from build123d import *

# Parameters (mm, degrees)
SKETCH_1_W             = 40
SKETCH_1_H             = 58
EXTRUDE_2_DEPTH        = 36
SKETCH_2_W             = 36
SKETCH_2_H             = 13
CUT_EXTRUDE_1_DEPTH    = 36
SKETCH_3_W             = 16
SKETCH_3_H             = 32
CUT_EXTRUDE_2_DEPTH    = 36
CUT_EXTRUDE_3_DEPTH    = 5
HOLE_WIZARD_M6_1_D     = 5
HOLE_WIZARD_M6_1_DEPTH = 15
HOLE_WIZARD_M6_1_TIP   = 1.502151548
CUT_EXTRUDE_START      = -36
SKETCH_8_W             = 12
SKETCH_8_H             = 32
CUT_EXTRUDE_4_DEPTH    = 36
FILLET_1_R             = 3
FILLET_2_R             = 5
SKETCH_9_W             = 36
SKETCH_9_H             = 32
CUT_EXTRUDE_5_DEPTH    = 0.5


with BuildPart() as part:
    # 草图1 → 凸台-拉伸2 (new body)
    with BuildSketch(Plane.XY):
        with Locations((20, 29)):
            Rectangle(SKETCH_1_W, SKETCH_1_H)
    extrude(amount=EXTRUDE_2_DEPTH)

    # 草图2 → 切除-拉伸1 (cut)
    with BuildSketch(Plane.ZY):
        with Locations((18, 51.5)):
            Rectangle(SKETCH_2_W, SKETCH_2_H)
        with Locations((18, 6.5)):
            Rectangle(SKETCH_2_W, SKETCH_2_H)
    extrude(amount=-CUT_EXTRUDE_1_DEPTH, mode=Mode.SUBTRACT)

    # 草图3 → 切除-拉伸2 (cut)
    with BuildSketch(Plane.ZY):
        with Locations((28, 29)):
            Rectangle(SKETCH_3_W, SKETCH_3_H)
    extrude(amount=-CUT_EXTRUDE_2_DEPTH, mode=Mode.SUBTRACT)

    # 草图4 → 切除-拉伸3 (cut)
    with BuildSketch(Plane(origin=(40, 0, 0), x_dir=(0, 0, -1), z_dir=(1, 0, 0))):
        with BuildLine():
            Line((-29, 53.1), (-7, 53.1))
            ThreePointArc((-7, 53.1), (-4.9, 51), (-7, 48.9))
            Line((-7, 48.9), (-29, 48.9))
            ThreePointArc((-29, 48.9), (-31.1, 51), (-29, 53.1))
        make_face()
        with BuildLine():
            Line((-29, 9.1), (-7, 9.1))
            ThreePointArc((-7, 9.1), (-4.9, 7), (-7, 4.9))
            Line((-7, 4.9), (-29, 4.9))
            ThreePointArc((-29, 4.9), (-31.1, 7), (-29, 9.1))
        make_face()
    extrude(amount=-CUT_EXTRUDE_3_DEPTH, mode=Mode.SUBTRACT)

    # M6 螺纹孔1
    with Locations(Plane.XY.offset(20)):
        with Locations((26, 29), (8, 29)):
            Hole(HOLE_WIZARD_M6_1_D / 2, depth=HOLE_WIZARD_M6_1_DEPTH)
            with Locations((0, 0, -(HOLE_WIZARD_M6_1_DEPTH + HOLE_WIZARD_M6_1_TIP / 2))):  # 118° drill point
                Cone(0, HOLE_WIZARD_M6_1_D / 2, HOLE_WIZARD_M6_1_TIP, mode=Mode.SUBTRACT)

    # 草图8 → 切除-拉伸4 (cut)
    with BuildSketch(Plane.ZY.offset(CUT_EXTRUDE_START)):
        with Locations((6, 29)):
            Rectangle(SKETCH_8_W, SKETCH_8_H)
    extrude(amount=CUT_EXTRUDE_4_DEPTH, mode=Mode.SUBTRACT)

    # 圆角1
    fillet_1_edges = [part.edges().sort_by_distance(p)[0] for p in [
        (38, 58, 36),
        (38, 0, 0),
        (38, 0, 36),
        (38, 58, 0),
    ]]
    fillet(fillet_1_edges, radius=FILLET_1_R)

    # 圆角2
    fillet_2_edges = [part.edges().sort_by_distance(p)[0] for p in [
        (0, 45, 16),
        (0, 13, 16),
    ]]
    fillet(fillet_2_edges, radius=FILLET_2_R)

    # 草图9 → 切除-拉伸5 (cut)
    with BuildSketch(Plane(origin=(40, 0, 0), x_dir=(0, 0, -1), z_dir=(1, 0, 0))):
        with Locations((-18, 29)):
            Rectangle(SKETCH_9_W, SKETCH_9_H)
    extrude(amount=-CUT_EXTRUDE_5_DEPTH, mode=Mode.SUBTRACT)


solid = part.part
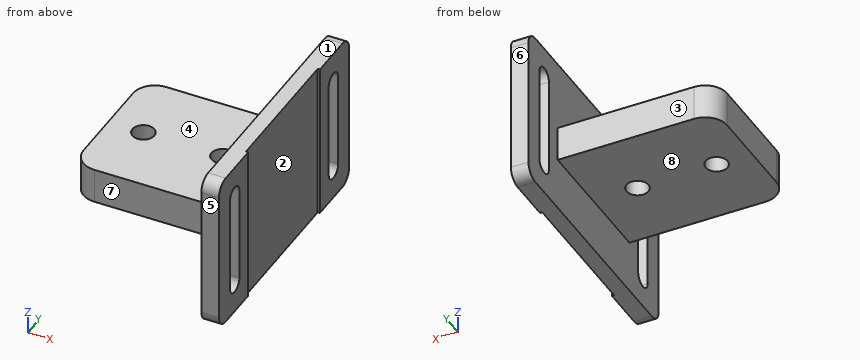
Source: CAD feature listing. Evaluate the final solid. Frame: model axes, mm. Face numbers are marked on the shaded views. A direction names the side the tool comes from. Coordinates: 2 decimals unless noted, no trailing zeros. Loops run counter-clockwise (first coordinate to the right, second up) from the corner with the lowest first, then second, coordinate; pieces in that order, holes last. Notation, with made-up numbers: (-27, 46) - (11, 46) arc R10 cw to (11, 65) - close; hole circle Ø9 at (78.25, 45). An arc over 180 degrees is marked (long way). One line per item, written item: value. Start each with the question number.
1. Ray query, L1, parallel to Y at x = 8, z = 17; L2, parallel to Z at x = 20, y = 24; L3, parallel to X at y = 27, z = 22. Return the intervals inside material, ascending.
2. Set-up query: the marked faces 4, 5, 6, 7 and 8. Return all of +Z, -Z, +X, -X, +Y, -Y with unobstructed straight access to the full face (end or side cutting, diameter ignored); none if empty.
3. Section C-C (y = 7). Return the cut outline in (x, z).
4. Section B-B (y = 29). Return the cut outline in (x, z).
5. Section D-D (y = 39). Return the cut outline in (x, z), and give its area (3 significant figures).
6. Mould query, pull axis Y, two halves, no side actions, for the marked faces 1, 2 and 3. Classes: pulls with the +Y half, pulls with the -Y half, needs draft (parallel to the pull), parting line crosses it, or undercut.
7. Contact query for flat-ended pins moving along their axis: P1, Ø1.5, axis at y = 30.5, z = 13, coming from the +X side; P2, Ø12, axis at y = 25, z = 26.5, coming from the -X side; P3, Ø6, axis at x = 8, y = 29, coming from the -Z side. Output: stop coordinate, or through.
8. Section A-A (x = 26). Return the cut outline in (y, z).
Verdict:
1. L1: y = 13 to 26.5, 31.5 to 45
1. L2: z = 12 to 20
1. L3: x = 36 to 39.5
2. face 4: +Z, -X, +Y, -Y
2. face 5: +Z, -Z, +X, -X, -Y
2. face 6: +Z, -Z, +X, -X, +Y
2. face 7: +Z, -Z, -X, -Y
2. face 8: -Z, -X, +Y, -Y
3. outline: (36, 0) - (40, 0) - (40, 4.9) - (36, 4.9) - close; (36, 31.1) - (40, 31.1) - (40, 36) - (36, 36) - close
4. outline: (0, 12) - (5.5, 12) - (5.5, 20) - (0, 20) - close; (10.5, 12) - (23.5, 12) - (23.5, 20) - (10.5, 20) - close; (28.5, 12) - (36, 12) - (36, 0) - (39.5, 0) - (39.5, 36) - (36, 36) - (36, 20) - (28.5, 20) - close
5. outline: (0, 12) - (36, 12) - (36, 0) - (39.5, 0) - (39.5, 36) - (36, 36) - (36, 20) - (0, 20) - close
5. area: 414 mm2
6. face 1: needs draft
6. face 2: undercut
6. face 3: pulls with the +Y half
7. P1: stops at x = 39.5
7. P2: stops at x = 36
7. P3: stops at z = 12
8. outline: (13, 12) - (26.5, 12) - (26.5, 20) - (13, 20) - close; (31.5, 12) - (45, 12) - (45, 20) - (31.5, 20) - close
